from build123d import *

# Parameters (mm, degrees)
F1_DEPTH  = 50
F2_R      = 1.5
F3_DEPTH  = 6.001
F4_DEPTH  = 3
F5_R      = 1
F6_DEPTH  = 5.001
F5_R_2    = 3
F7_DEPTH  = 2
F9_DEPTH  = 25
F10_R     = 1
F11_DEPTH = 18.001


with BuildPart() as f1:
    # F0 (on Right) → F1 (new body)
    with BuildSketch(Plane.YZ):
        Polygon((6, 5), (6, 25), (0, 25), (0, 0), (34, 0), (34, 25), (30, 25), (30, 5), align=None)
    extrude(amount=F1_DEPTH)

    # F2 (on face) → F3 (cut, through all)
    with BuildSketch(Plane(origin=(0, 6, 0), x_dir=(-1, 0, 0), z_dir=(0, 1, 0))):
        with Locations((-40, 13)):
            Circle(F2_R)
        with Locations((-12, 13)):
            Circle(F2_R)
    extrude(amount=-F3_DEPTH, mode=Mode.SUBTRACT)

    # F2 (on face) → F4 (cut, through all)
    with BuildSketch(Plane(origin=(0, 6, 0), x_dir=(-1, 0, 0), z_dir=(0, 1, 0))):
        Polygon((-41.5877132403, 15.75), (-43.1754264805, 13), (-41.5877132403, 10.25), (-38.4122867597, 10.25), (-36.8245735195, 13), (-38.4122867597, 15.75), align=None)
        with Locations((-40, 13)):
            Circle(F2_R, mode=Mode.SUBTRACT)
        Polygon((-13.5877132403, 15.75), (-15.1754264805, 13), (-13.5877132403, 10.25), (-10.4122867597, 10.25), (-8.8245735195, 13), (-10.4122867597, 15.75), align=None)
        with Locations((-12, 13)):
            Circle(F2_R, mode=Mode.SUBTRACT)
    extrude(amount=-F4_DEPTH, mode=Mode.SUBTRACT)

    # F5 (on face) → F6 (cut, through all)
    with BuildSketch(Plane.XY.offset(5)):
        with Locations((8.5, 14)):
            Circle(F5_R)
        with Locations((41.5, 25.5)):
            Circle(F5_R)
    extrude(amount=-F6_DEPTH, mode=Mode.SUBTRACT)

    # F5 (on face) → F7 (join)
    with BuildSketch(Plane.XY.offset(5)):
        with Locations((8.5, 14)):
            Circle(F5_R_2)
        with Locations((8.5, 14)):
            Circle(F5_R, mode=Mode.SUBTRACT)
        with Locations((41.5, 25.5)):
            Circle(F5_R_2)
        with Locations((41.5, 25.5)):
            Circle(F5_R, mode=Mode.SUBTRACT)
    extrude(amount=F7_DEPTH)

    # F8 (on face) → F9 (join)
    with BuildSketch(Plane.YZ.offset(50)):
        Polygon((48, 18), (34, 18), (34, 14), (44, 14), (44, 0), (48, 0), align=None)
    extrude(amount=-F9_DEPTH)

    # F10 (on face) → F11 (cut, through all)
    with BuildSketch(Plane.XY.offset(18)):
        with Locations((37.5, 39)):
            Circle(F10_R)
    extrude(amount=-F11_DEPTH, mode=Mode.SUBTRACT)


solid = f1.part
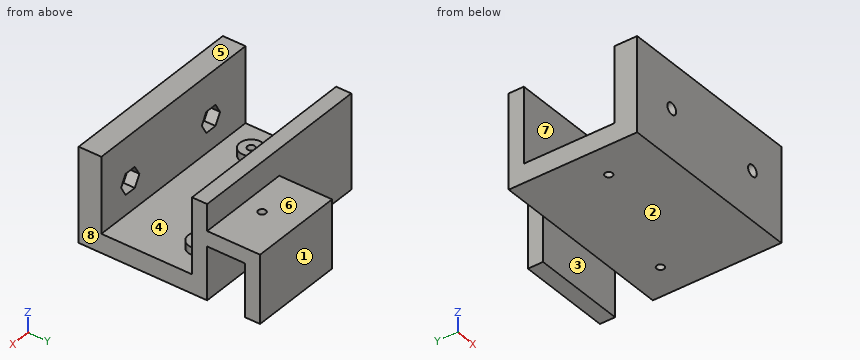
The model under review builds one solid part; all positions refer to its coordinate system, in mm. Face numbers are marked on the shaded views. A direction names the side the tool comes from. Round coordinates to 2 decimals unless told otherwise and drop trailing zeros. Write each loop counter-clockwise with the first axis right and the second up, starting at its lowest first coordinate (ties: lowest second). Pieces come first, ordered by that corner, then holes. Notation, with made-up numbers: M 22,88 L 43,88 A27 cw 43,126 Z; hole C 24.25,66 d9. An arc over 180 degrees is marked long. Answer as CSV lines item,"result". Start each with the question number.
Q1. Tool access review of the marked faces 4, 5, 6, 7 and 8: name each direction out of +Z, -Z, +X, -X, +Y, -Y from which nothing blocks a thin tool from reaching the whole face with its end or side.
Q2. Wall thickness on line 1 along Y through (x, z) = (41.5, 6.3); line 2 along Y through (x, z) = (8.5, 5.85); line 3 along Y through (x, z) = (37.5, 17.2): over which ranges is each line inside the solid? List them lowest first.
Q3. The part is to be moulded in two halves that separate along Y. For the marked faces 1, 2 and 3, say which applies: +Y half, -Y half, draft (parallel to the pull), parting line (faces both ways), or undercut.
Q4. Consider section D-D, the plane x = 20. Give the boundary of the cut face in (y, z).
Q5. Consider section C-C, the plane y = 39. Give the boundary of the cut face in (x, z), then the cut area to 3 significant figures.
Q6. Clearance check with flat-ended pins moving along their axes: P1, Ø2, axis at x = 25.5, y = 26.5, coming from the +Z side; P2, Ø4, axis at y = 44, z = 5, coming from the -X side; P3, Ø5, axis at x = 9, y = 13.5, coming from the +Z side; P4, Ø1.2, axis at x = 37.5, y = 39, coming from the +Z side. State where each tip first meets the part, or that it passes through.
Q7. Consider section A-A, the plane z = 8. Give the boundary of the cut face in (x, y), then the cut area to 3 significant figures.
Q8. Consider section B-B, the plane z = 2.75. Give the boundary of the cut face in (x, y).
Result set:
1,face 4,"+Z"
1,face 5,"+Z, +X, -X, +Y, -Y"
1,face 6,"+Z, +X, -X, +Y"
1,face 7,"+Z, +X, -X"
1,face 8,"+Z, -Z, +X, +Y, -Y"
2,line 1,"y = 0 to 6, 22.5 to 24.5, 26.5 to 28.5, 30 to 34, 44 to 48"
2,line 2,"y = 0 to 6, 11 to 13, 15 to 17, 30 to 34"
2,line 3,"y = 0 to 6, 30 to 38, 40 to 48"
3,face 1,"+Y half"
3,face 2,"draft"
3,face 3,"undercut"
4,outline,"M 0,0 L 34,0 L 34,25 L 30,25 L 30,5 L 6,5 L 6,25 L 0,25 Z"
5,outline,"M 25,14 L 36.5,14 L 36.5,18 L 25,18 Z; M 38.5,14 L 50,14 L 50,18 L 38.5,18 Z"
5,area,"92.0 mm²"
6,P1,"stops at z = 5"
6,P2,"stops at x = 25"
6,P3,"stops at z = 7"
6,P4,"passes through"
7,outline,"M 0,0 L 50,0 L 50,6 L 0,6 Z; M 0,30 L 50,30 L 50,34 L 0,34 Z; M 25,44 L 50,44 L 50,48 L 25,48 Z"
7,area,"600 mm²"
8,outline,"M 0,0 L 50,0 L 50,34 L 0,34 Z; M 25,44 L 50,44 L 50,48 L 25,48 Z; hole C 8.5,14 d2; hole C 41.5,25.5 d2"
